Build history of the part. All positions in model axes, mm. A direction names the side the tool comes from. Coordinates: 2 decimals unless noted, no trailing zeros. Write each loop counter-clockwise with the first axis right and the second up, starting at its lowest first coordinate (ties: lowest second). Pieces come first, ordered by that corner, then holes.
```python
from build123d import *

# Parameters (mm, degrees)
SKETCH_R        = 1.8
PAD_DEPTH       = 20
POCKET_DEPTH    = 10
SKETCH002_W     = 4
SKETCH002_H     = 8
PAD001_DEPTH    = 10
SKETCH003_R     = 1.4
POCKET001_DEPTH = 5


with BuildPart() as part:
    # Sketch → Pad (new body)
    with BuildSketch(Plane.YZ):
        with BuildLine():
            ThreePointArc((0, 10), (-5, 5), (0, 0))
            Line((0, 0), (100, 0))
            Line((100, 0), (100, 10))
            Line((100, 10), (0, 10))
        make_face()
        with Locations((0, 5)):
            Circle(SKETCH_R, mode=Mode.SUBTRACT)
    extrude(amount=PAD_DEPTH)

    # Sketch001 → Pocket (cut)
    with BuildSketch(Plane.XY.offset(10)):
        with BuildLine():
            ThreePointArc((11.7, 95), (10, 96.7), (8.3, 95))
            Line((8.3, 15), (8.3, 95))
            ThreePointArc((8.3, 15), (10, 13.3), (11.7, 15))
            Line((11.7, 95), (11.7, 15))
        make_face()
    extrude(amount=-POCKET_DEPTH, mode=Mode.SUBTRACT)

    # Sketch002 → Pad001 (new body)
    with BuildSketch(Plane(origin=(0, 0, 0), x_dir=(1, 0, 0), z_dir=(0, 0, -1))):
        with Locations((2, -19)):
            Rectangle(SKETCH002_W, SKETCH002_H)
        with Locations((2, -50)):
            Rectangle(SKETCH002_W, SKETCH002_H)
    extrude(amount=PAD001_DEPTH)

    # Sketch003 → Pocket001 (cut)
    with BuildSketch(Plane(origin=(0, 0, 0), x_dir=(0, -1, 0), z_dir=(-1, 0, 0))):
        with Locations((-48.5, -6)):
            Circle(SKETCH003_R)
        with Locations((-20.5, -6)):
            Circle(SKETCH003_R)
    extrude(amount=-POCKET001_DEPTH, mode=Mode.SUBTRACT)


solid = part.part
```
1. Mould opens along X. For faces 4 (the face through (10, 100, 5)), 5 (the face through (10, 96.7, 5.1)), 6 (the face through (20, 47, 5)), 7 (the face through (8.3, 54, 5)) say: +X half, -X half, draft (parallel to the pull), parting line (faces both ways), or undercut.
Computed values:
face 4: draft
face 5: undercut
face 6: +X half
face 7: undercut
2. Flat gauge pins, fed straight in: pin 1 (1 mm diameter, centred on x = 5.5, y = 47, fed in from -Z); pin 2 (4 mm diameter, centred on y = 50.5, z = -5, fed in from +X); pin 3 (1.2 mm diameter, centred on x = 1.5, z = -7, fed in from +Y). Where does each tip first touch, or does it go through?
Computed values:
pin 1: stops at z = 0
pin 2: stops at x = 4
pin 3: stops at y = 54
3. 3-axis set-ups, long thin cutter, end or side, ignore diameter. For faces 1 (the face through (4, 19, -5)), 2 (the face through (10, 13.3, 5.1)), 3 (the face through (2, 54, -5)): which of +Z, -Z, +X, -X, +Y, -Y reach the whole face in a straight line?
Computed values:
face 1: -Z, +X, +Y, -Y
face 2: +Z, -Z
face 3: -Z, +X, -X, +Y
4. Saw through at C-C on y = 20.5. List the corners of the cut face in (x, z).
Computed values:
outline: (0, -10) - (4, -10) - (4, -7.4) - (0, -7.4) - close; (0, -4.6) - (4, -4.6) - (4, 0) - (8.3, 0) - (8.3, 10) - (0, 10) - close; (11.7, 0) - (20, 0) - (20, 10) - (11.7, 10) - close
5. Saw through at D-D on z = -6. List the corners of the cut face in (x, y), plus the area to 3 significant figures.
Computed values:
outline: (0, 15) - (4, 15) - (4, 19.1) - (0, 19.1) - close; (0, 21.9) - (4, 21.9) - (4, 23) - (0, 23) - close; (0, 46) - (4, 46) - (4, 47.1) - (0, 47.1) - close; (0, 49.9) - (4, 49.9) - (4, 54) - (0, 54) - close
area: 41.6 mm2
6. Saw through at A-A on z = 5. List the corners of the cut face in (x, y).
Computed values:
outline: (0, -5) - (20, -5) - (20, -1.8) - (0, -1.8) - close; (0, 1.8) - (20, 1.8) - (20, 100) - (0, 100) - close; hole (8.3, 15) arc R1.7 ccw to (11.7, 15) - (11.7, 95) arc R1.7 ccw to (8.3, 95) - close
7. Saw through at B-B on y = 35.5. List the corners of the cut face in (x, z), plus the area to 3 significant figures.
Computed values:
outline: (0, 0) - (8.3, 0) - (8.3, 10) - (0, 10) - close; (11.7, 0) - (20, 0) - (20, 10) - (11.7, 10) - close
area: 166 mm2
8. Probe line 1 along X through (y, z) = (89.5, 6); line 2 along Z through (x, y) = (15, 0); line 3 along Z through (x, y) = (1.6, 20.5). List the from-to ranges inside material, lowest first.
Computed values:
line 1: x = 0 to 8.3, 11.7 to 20
line 2: z = 0 to 3.2, 6.8 to 10
line 3: z = -10 to -7.4, -4.6 to 10
